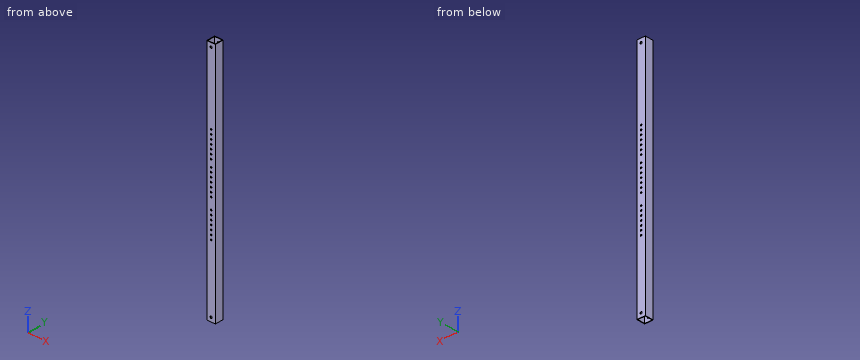
```python
from build123d import *

# Parameters (mm, degrees)
SKETCH1_W            = 25.4
SKETCH1_H            = 25.4
SKETCH1_W_2          = 22.225
SKETCH1_H_2          = 22.225
BOSS_EXTRUDE1_DEPTH  = 357.759
SKETCH2_R            = 2.38125
CUT_EXTRUDE1_DEPTH   = 26.4
SKETCH3_R            = 2.38125
CUT_EXTRUDE2_DEPTH   = 26.4
M6_CLEARANCE_HOLE1_D = 6.6


with BuildPart() as part:
    # Sketch1 → Boss-Extrude1 (new body, symmetric)
    with BuildSketch(Plane.XY):
        Rectangle(SKETCH1_W, SKETCH1_H)
        Rectangle(SKETCH1_W_2, SKETCH1_H_2, mode=Mode.SUBTRACT)
    extrude(amount=BOSS_EXTRUDE1_DEPTH, both=True)

    # Sketch2 → Cut-Extrude1 (cut, through all)
    with BuildSketch(Plane.XZ.offset(12.7)):
        with Locations((0, -37.973)):
            Circle(SKETCH2_R)
        with Locations((0, -25.273)):
            Circle(SKETCH2_R)
        with Locations((0, -12.573)):
            Circle(SKETCH2_R)
        with Locations((0, 0.127)):
            Circle(SKETCH2_R)
        with Locations((0, 12.827)):
            Circle(SKETCH2_R)
        with Locations((0, 25.527)):
            Circle(SKETCH2_R)
        with Locations((0, 38.227)):
            Circle(SKETCH2_R)
    extrude(amount=-CUT_EXTRUDE1_DEPTH, mode=Mode.SUBTRACT)

    # Sketch3 → Cut-Extrude2 (cut, through all)
    with BuildSketch(Plane.XZ.offset(12.7)):
        with Locations((0, 59.018644472)):
            Circle(SKETCH3_R)
        with Locations((0, 71.718644472)):
            Circle(SKETCH3_R)
        with Locations((0, 84.418644472)):
            Circle(SKETCH3_R)
        with Locations((0, 109.818644472)):
            Circle(SKETCH3_R)
        with Locations((0, 122.518644472)):
            Circle(SKETCH3_R)
        with Locations((0, 135.218644472)):
            Circle(SKETCH3_R)
        with Locations((0, 97.118644472)):
            Circle(SKETCH3_R)
        with Locations((0, -71.18135497)):
            Circle(SKETCH3_R)
        with Locations((0, -83.88135497)):
            Circle(SKETCH3_R)
        with Locations((0, -96.58135497)):
            Circle(SKETCH3_R)
        with Locations((0, -109.28135497)):
            Circle(SKETCH3_R)
        with Locations((0, -121.98135497)):
            Circle(SKETCH3_R)
        with Locations((0, -134.68135497)):
            Circle(SKETCH3_R)
        with Locations((0, -147.38135497)):
            Circle(SKETCH3_R)
    extrude(amount=-CUT_EXTRUDE2_DEPTH, mode=Mode.SUBTRACT)

    # M6 Clearance Hole1 (through all)
    with Locations(Plane(origin=(0, -12.7, 0), x_dir=(-1, 0, 0), z_dir=(0, -1, 0))):
        with Locations((0, -345.759), (0, 345.759)):
            Hole(M6_CLEARANCE_HOLE1_D / 2)


solid = part.part
```
Geometry: final body of the model. Coordinates: model frame, mm. Give positions to 0.01 mm unless a question says otherwise; leave off trailing zeros. Loops run counter-clockwise (first coordinate to the right, second up) from the corner with the lowest first, then second, coordinate; pieces in that order, holes last. Notation, with made-up numbers: (71, 33) -> (80, 33) arc R19 cw to (80, 43) -> close; hole circle Ø9 at (-32, -33). An arc over 180 degrees is marked (long way). Return JSON: item names as keys, results as strings.
Item 1: Section A-A, the plane y = -1.25. Output: boundary loops of the cut face in (x, z), plus the area to 3 significant figures.
Filled in:
{"outline": "(-12.7, -357.76) -> (-11.11, -357.76) -> (-11.11, 357.76) -> (-12.7, 357.76) -> close; (11.11, -357.76) -> (12.7, -357.76) -> (12.7, 357.76) -> (11.11, 357.76) -> close", "area": "2,270 mm^2"}
Item 2: Section B-B, the plane z = 258. Output: boundary loops of the cut face in (x, y).
Filled in:
{"outline": "(-12.7, -12.7) -> (12.7, -12.7) -> (12.7, 12.7) -> (-12.7, 12.7) -> close; hole (-11.11, -11.11) -> (11.11, -11.11) -> (11.11, 11.11) -> (-11.11, 11.11) -> close"}
Item 3: Line query: line 1 (Y direction, x = -0.5, z = -161). Output: solid intervals per line, ascending.
Filled in:
{"line 1": "-12.7 to -11.11, 11.11 to 12.7"}
